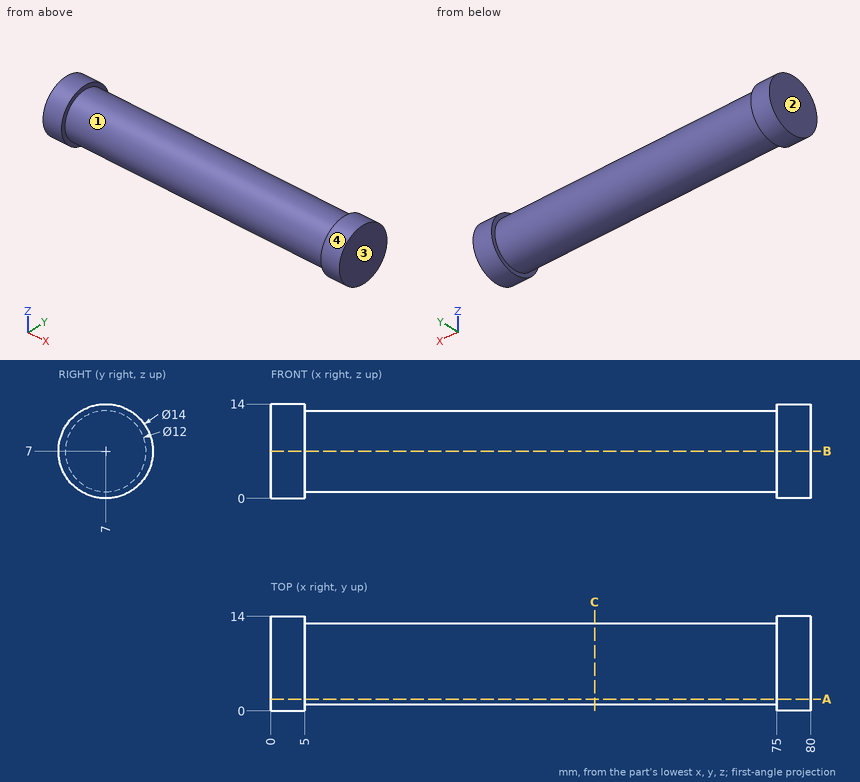
Source: three-view drawing plus pictorial views. Frame: mm from the lowest corner of the part. Round coordinates to 2 decimals unless told otherwise and drop trailing zeros. Loops run counter-clockwise (first coordinate to the right, second up) from the corner with the lowest first, then second, coordinate; pieces in that order, holes last.
1. Section query C-C on x = 48. Output: boundary loops of the cut face in (y, z), and give its area (3 significant figures).
2. Section query B-B on z = 7. Output: boundary loops of the cut face in (x, y).
3. Contact query for flat-ended pins moving along their axis: pin 1 (1 mm diameter, centred on x = 31, y = 6, fed in from +Z); pin 2 (1 mm diameter, centred on x = 17, z = 2.5, fed in from +Y); pin 3 (8 mm diameter, centred on x = 39, y = 6, fed in from -Z). Output: stop coordinate, or through.
4. Ray query, L1, parallel to X at y = 10, z = 12.5; L2, parallel to Z at x = 28, y = 6.75; L3, parallel to Y at x = 44, z = 2. Return the intervals inside material, ascending.
5. Section query A-A on y = 1.75. Output: boundary loops of the cut face in (x, z), and give its area (3 significant figures).
6. Mould query, pull axis X, two halves, no side actions, for the marked faces 1, 2, 3 and 4. Classes: released by +X, released by -X, zero draft, split by the parting line, or undercut.
Answers below:
1. outline: circle Ø12 at (7, 7)
1. area: 113 mm2
2. outline: (0, 0) - (5, 0) - (5, 1) - (75, 1) - (75, 0) - (80, 0) - (80, 14) - (75, 14) - (75, 13) - (5, 13) - (5, 14) - (0, 14) - close
3. pin 1: stops at z = 12.98
3. pin 2: stops at y = 11.47
3. pin 3: stops at z = 1
4. L1: x = 0 to 5, 75 to 80
4. L2: z = 1.01 to 12.99
4. L3: y = 3.68 to 10.32
5. outline: (0, 2.37) - (5, 2.37) - (5, 4.1) - (75, 4.1) - (75, 2.37) - (80, 2.37) - (80, 11.63) - (75, 11.63) - (75, 9.9) - (5, 9.9) - (5, 11.63) - (0, 11.63) - close
5. area: 499 mm2
6. face 1: undercut
6. face 2: released by -X
6. face 3: released by +X
6. face 4: zero draft
